from build123d import *

# Parameters (mm, degrees)
F0_W     = 21.25
F0_H     = 15.36
F1_DEPTH = 8
F2_T     = -2
F3_W     = 4
F3_H     = 1
F4_DEPTH = 1
F5_W     = 4
F5_H     = 1
F6_DEPTH = 1


# Not quite as in the source:
# - a feature names something its author has since deleted; it is built from what else it names


with BuildPart() as f1:
    # F0 (on Top) → F1 (new body)
    with BuildSketch(Plane.XY):
        Rectangle(F0_W, F0_H)
    extrude(amount=F1_DEPTH)

    # F2
    f2_openings = [f1.faces().sort_by_distance(p)[0] for p in [
        (0, 0, 8),
    ]]
    offset(amount=F2_T, openings=f2_openings)

    # F3 (on face) → F4 (join)
    with BuildSketch(Plane(origin=(-10.625, 0, 0), x_dir=(0, -1, 0), z_dir=(-1, 0, 0))):
        with Locations((0, 0.5)):
            Rectangle(F3_W, F3_H)
    extrude(amount=F4_DEPTH)

    # F5 (on face) → F6 (join)
    with BuildSketch(Plane.YZ.offset(10.625)):
        with Locations((0, 0.5)):
            Rectangle(F5_W, F5_H)
    extrude(amount=F6_DEPTH)


solid = f1.part
Read the model definition and answer for the solid it produces. Units are mm, in the model's axes. A direction names the side the tool comes from. Give positions to 0.01 mm unless a question says otherwise; leave off trailing zeros. Write each loop counter-clockwise with the first axis right and the second up, starting at its lowest first coordinate (ties: lowest second). Pieces come first, ordered by that corner, then holes. Notation, with made-up numbers: (8, 29.5) - (39, 29.5) arc R16 ccw to (39, 49.5) - close; hole circle Ø9 at (6, 73.5). An arc over 180 degrees is marked (long way). Return JSON: item names as keys, results as strings.
Q1. For a pull along Y with two mould halves and no side action, classify faces 4 (the face through (11.1, -2, 0.5)), 5 (the face through (0, 0, 2)), 6 (the face through (11.625, 0, 0.5)), 7 (the face through (8.625, 0, 5)) as released by +Y, released by -Y, zero draft, split by the parting line, or undercut.
Reply:
{"face 4": "released by -Y", "face 5": "undercut", "face 6": "zero draft", "face 7": "undercut"}
Q2. A cutting plane is placed at B-B, the plane y = 5. Determine the outline of the cut face in (x, z) (3 decimals), and give its area (3 significant figures).
Reply:
{"outline": "(-10.625, 0) - (10.625, 0) - (10.625, 8) - (8.625, 8) - (8.625, 2) - (-8.625, 2) - (-8.625, 8) - (-10.625, 8) - close", "area": "66.5 mm²"}
Q3. A cutting plane is placed at A-A, the plane z = 2.75. Determine the outline of the cut face in (x, y) (3 decimals).
Reply:
{"outline": "(-10.625, -7.68) - (10.625, -7.68) - (10.625, 7.68) - (-10.625, 7.68) - close; hole (-8.625, -5.68) - (8.625, -5.68) - (8.625, 5.68) - (-8.625, 5.68) - close"}
Q4. A cutting plane is placed at D-D, the plane y = 1.75. Determine the outline of the cut face in (x, z) (3 decimals), and give its area (3 significant figures).
Reply:
{"outline": "(-11.625, 0) - (11.625, 0) - (11.625, 1) - (10.625, 1) - (10.625, 8) - (8.625, 8) - (8.625, 2) - (-8.625, 2) - (-8.625, 8) - (-10.625, 8) - (-10.625, 1) - (-11.625, 1) - close", "area": "68.5 mm²"}
Q5. A cutting plane is placed at C-C, the plane x = -0.5. Determine the outline of the cut face in (y, z), and give its area (3 significant figures).
Reply:
{"outline": "(-7.68, 0) - (7.68, 0) - (7.68, 8) - (5.68, 8) - (5.68, 2) - (-5.68, 2) - (-5.68, 8) - (-7.68, 8) - close", "area": "54.7 mm²"}
Q6. Given P1, Ø1.5, axis at x = -2.5, y = 3, coming from the -Z side; P2, Ø0.5, axis at x = 11, z = 0.5, coming from the +Y side; P3, Ø3, axis at y = 1, z = 6, coming from the -X side (3 decimals); P4, Ø2.5, axis at y = 1, z = 4, coming from the +X side (3 decimals), each flat-ended and moving along its own axis, determine where each tip first touches the part or whether it passes through.
Reply:
{"P1": "z = 0", "P2": "y = 2", "P3": "x = -10.625", "P4": "x = 10.625"}
Q7. For faces 1 (the face through (0, -5.68, 5)), 2 (the face through (11.1, 2, 0.5)), 3 (the face through (11, 0, 1)), determine the directions among +Z, -Z, +X, -X, +Y, -Y from which every point of the face is accessible in a straight line to the end or side of a thin tool.
Reply:
{"face 1": "+Z", "face 2": "+Z, -Z, +X, +Y", "face 3": "+Z, +X, +Y, -Y"}
Q8. Consider line 1 along X through (y, z) = (-2.5, 7.75) (3 decimals); line 2 along Y through (x, z) = (-6.5, 6); line 3 along X through (y, z) = (-5.75, 5) (3 decimals). Determine where each line is inside the solid, lowest interval first. Write a range as [from, to].
Reply:
{"line 1": "[-10.625, -8.625], [8.625, 10.625]", "line 2": "[-7.68, -5.68], [5.68, 7.68]", "line 3": "[-10.625, 10.625]"}
